```python
from build123d import *

# Parameters (mm, degrees)
F0_R     = 3.175
F1_DEPTH = 3.048


with BuildPart() as f1:
    # F0 (on Front) → F1 (new body)
    with BuildSketch(Plane.XZ):
        with BuildLine():
            ThreePointArc((0.6773435479, -9.500885786), (6.9705567315, -6.4912990883), (9.525, 0))
            ThreePointArc((9.525, 0), (0, 9.525), (-9.525, 0))
            ThreePointArc((-9.525, 0), (-6.7351920908, -6.7351920908), (0, -9.525))
            Line((0, -9.525), (0.6773435479, -9.500885786))
        make_face()
        Circle(F0_R, mode=Mode.SUBTRACT)
        with BuildLine():
            ThreePointArc((-9.525, 0), (0, 9.525), (9.525, 0))
            ThreePointArc((9.525, 0), (6.9705567315, -6.4912990883), (0.6773435479, -9.500885786))
            Line((0.6773435479, -9.500885786), (44.7324052746, -7.9324746146))
            ThreePointArc((44.7324052746, -7.9324746146), (36.5137564458, -0.1412249921), (44.45, 7.9375))
            Line((44.45, 7.9375), (18.6544621675, 12.4908351229))
            ThreePointArc((18.6544621675, 12.4908351229), (13.7263384996, 15.4838524031), (12.1171642333, 21.020558419))
            Line((12.1171642333, 21.020558419), (15.6284662769, 60.7131259747))
            ThreePointArc((15.6284662769, 60.7131259747), (0.1815405689, 47.626038049), (-15.5606435644, 60.3564356436))
            Line((-15.5606435644, 60.3564356436), (-9.525, 0))
        make_face()
        with BuildLine():
            ThreePointArc((0, -9.525), (0.3388863295, -9.5189695375), (0.6773435479, -9.500885786))
            Line((0.6773435479, -9.500885786), (0, -9.525))
        make_face()
        with BuildLine():
            Line((-15.875, 63.5), (-15.5606435644, 60.3564356436))
            ThreePointArc((-15.5606435644, 60.3564356436), (0.1815405689, 47.626038049), (15.6284662769, 60.7131259747))
            Line((15.6284662769, 60.7131259747), (15.875, 63.5))
            Line((15.875, 63.5), (15.3865384615, 67.4076923077))
            ThreePointArc((15.3865384615, 67.4076923077), (0, 79.375), (-15.3865384615, 67.4076923077))
            Line((-15.3865384615, 67.4076923077), (-15.875, 63.5))
        make_face()
        with Locations((0, 63.5)):
            Circle(F0_R, mode=Mode.SUBTRACT)
        with BuildLine():
            ThreePointArc((-15.875, 63.5), (-15.7962153946, 61.9203784605), (-15.5606435644, 60.3564356436))
            Line((-15.5606435644, 60.3564356436), (-15.875, 63.5))
        make_face()
        with BuildLine():
            ThreePointArc((44.45, 7.9375), (36.5137564458, -0.1412249921), (44.7324052746, -7.9324746146))
            ThreePointArc((44.7324052746, -7.9324746146), (50.1616327839, -5.5119104847), (52.3875, 0))
            ThreePointArc((52.3875, 0), (50.0626600757, 5.6126600757), (44.45, 7.9375))
        make_face()
        with Locations((44.45, 0)):
            Circle(F0_R, mode=Mode.SUBTRACT)
        with BuildLine():
            ThreePointArc((-15.3865384615, 67.4076923077), (-15.7524112928, 65.4690514116), (-15.875, 63.5))
            Line((-15.875, 63.5), (-15.3865384615, 67.4076923077))
        make_face()
        with BuildLine():
            Line((15.875, 63.5), (15.6284662769, 60.7131259747))
            ThreePointArc((15.6284662769, 60.7131259747), (15.813246459, 62.1011213679), (15.875, 63.5))
        make_face()
        with BuildLine():
            Line((-9.525, 114.3), (-15.3865384615, 67.4076923077))
            ThreePointArc((-15.3865384615, 67.4076923077), (0, 79.375), (15.3865384615, 67.4076923077))
            Line((15.3865384615, 67.4076923077), (9.525, 114.3))
            ThreePointArc((9.525, 114.3), (0, 104.775), (-9.525, 114.3))
        make_face()
        with Locations((-1.5875, 100.0252)):
            Circle(F0_R, mode=Mode.SUBTRACT)
        with BuildLine():
            Line((15.3865384615, 67.4076923077), (15.875, 63.5))
            ThreePointArc((15.875, 63.5), (15.7524112928, 65.4690514116), (15.3865384615, 67.4076923077))
        make_face()
        with BuildLine():
            ThreePointArc((9.525, 114.3), (0, 123.825), (-9.525, 114.3))
            ThreePointArc((-9.525, 114.3), (0, 104.775), (9.525, 114.3))
        make_face()
        with Locations((0, 114.3)):
            Circle(F0_R, mode=Mode.SUBTRACT)
    extrude(amount=F1_DEPTH)


solid = f1.part
```
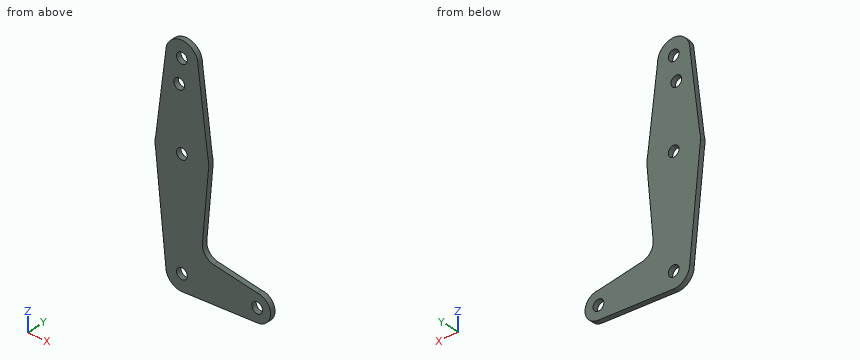
Geometry check sheet. Reference: the model listing, model coordinates, mm. Round coordinates to 2 decimals unless told otherwise and drop trailing zeros. Loops run counter-clockwise (first coordinate to the right, second up) from the corner with the lowest first, then second, coordinate; pieces in that order, holes last. Notation, with made-up numbers: M -5,-4.75 L 17,-4.75 A21 cw 17,22.25 Z; hole C -18.75,61.25 d11. An arc over 180 degrees is marked long. Return JSON: item names as keys, results as strings. Group by question number.
(1) Section check B-B, the plane x = 8. Enter the section's corners in (y, z), and give its area (3 significant figures).
(2) Go/stop test with a flat-tipped pin: pin 1 (12 mm diameter, centred on x = 18.5, z = 67.5, fed in from +Y). Record where the tip stops, or that it passes through.
(3) Section check A-A, the plane y = -2. Give the number of separate pieces and of enclosed holes in the cut face, and give its area (3 significant figures).
(4) Scan lines: line 1 along Z through (x, y) = (2.5, -2.15); line 2 along Z through (x, y) = (-1, -0.75); line 3 along Z through (x, y) = (-2, -1.65). Record each from-to range of solid material in increasing order. Write a range as [from, to].
(5) Section check C-C, the plane z = 24.5. Enter the section's corners in (x, y) (3 decimals).
Data:
{
 "1": {"outline": "M -3.05,-9.24 L 0,-9.24 L 0,119.47 L -3.05,119.47 Z", "area": "392 mm²"},
 "2": {"pin 1": "y = 0"},
 "3": {"separate pieces": "1", "enclosed holes": "5", "area": "3,850 mm²"},
 "4": {"line 1": "[-9.44, -1.96], [1.96, 61.54], [65.46, 112.34], [116.26, 123.49]", "line 2": "[-9.47, -3.01], [3.01, 60.49], [66.51, 96.91], [103.15, 111.29], [117.31, 123.77]", "line 3": "[-9.31, -2.47], [2.47, 61.03], [65.97, 96.88], [103.17, 111.83], [116.77, 123.61]"},
 "5": {"outline": "M -11.975,-3.048 L 12.425,-3.048 L 12.425,0 L -11.975,0 Z"}
}
